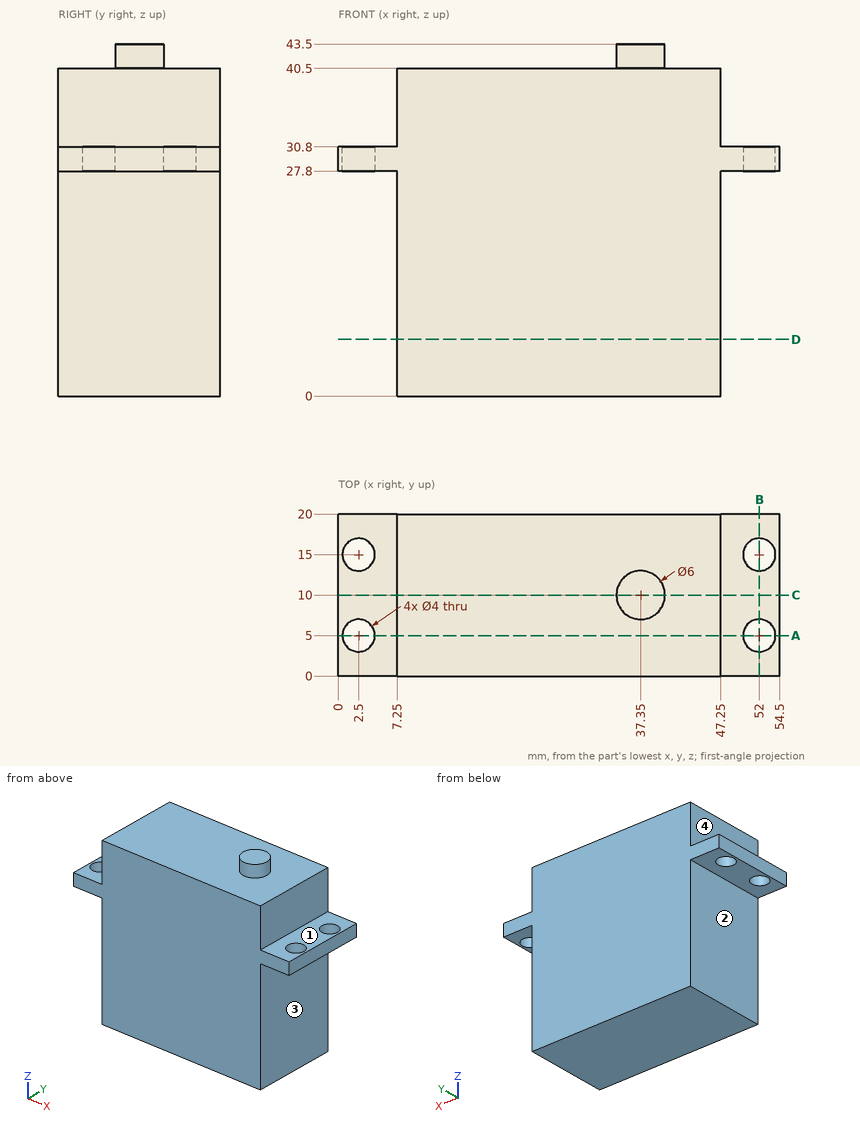
Could you check a few things on this drawing? It's one solid part, dimensions in mm from its lowest x, y, z. A direction names the side the tool comes from. Give positions to 0.01 mm unless a question says otherwise; leave off trailing zeros. Write each loop counter-clockwise with the first axis right and the second up, starting at its lowest first coordinate (ties: lowest second). Pieces come first, ordered by that corner, then holes. Notation, with made-up numbers: (39.5, 88) - (94.5, 88) arc R14 ccw to (94.5, 115) - close; hole circle Ø1 at (44.5, 70.5). An arc over 180 degrees is marked (long way). Use CSV: the item, a comma, the result in double quotes. Start each with the question number.
Item 1: I want a section at D-D, the plane z = 7. Please give me the cut outline in (x, y), then the cut area to 3 significant figures.
Item 2: If I drill on line 1 along Y through (x, z) = (2.5, 28.95); line 2 along Y through (x, z) = (2, 29); line 3 along X through (y, z) = (18, 34.5), over which ranges is the centre line in solid material (lowest first)?
Item 3: I want a section at C-C, the plane y = 10. Please give me the cut outline in (x, z), then the cut area to 3 significant figures.
Item 4: For the marked faces 1, 2, 3 and 4, which set-ups out of +Z, -Z, +X, -X, +Y, -Y let a thin tool reach every point of the face, with its end or its side?
Item 5: I want a section at A-A, the plane y = 5. Please give me the cut outline in (x, z).
Item 6: I'm going to push flat-ended pins straight in: pin 1 (3.5 mm diameter, centred on x = 52, y = 15, fed in from -Z); pin 2 (2 mm diameter, centred on y = 4, z = 17, fed in from -X); pin 3 (5 mm diameter, centred on x = 27, y = 14.5, fed in from +Z); pin 4 (4.5 mm diameter, centred on x = 2.5, y = 15, fed in from -Z). Where does each tip first touch, or does it pass through?
Item 7: I want a section at B-B, the plane x = 52. Please give me the cut outline in (y, z), then the cut area to 3 significant figures.
Findings:
1,outline,"(7.25, 0) - (47.25, 0) - (47.25, 20) - (7.25, 20) - close"
1,area,"800 mm2"
2,line 1,"y = 0 to 3, 7 to 13, 17 to 20"
2,line 2,"y = 0 to 3.06, 6.94 to 13.06, 16.94 to 20"
2,line 3,"x = 7.25 to 47.25"
3,outline,"(0, 27.8) - (7.25, 27.8) - (7.25, 0) - (47.25, 0) - (47.25, 27.8) - (54.5, 27.8) - (54.5, 30.8) - (47.25, 30.8) - (47.25, 40.5) - (40.35, 40.5) - (40.35, 43.5) - (34.35, 43.5) - (34.35, 40.5) - (7.25, 40.5) - (7.25, 30.8) - (0, 30.8) - close"
3,area,"1,680 mm2"
4,face 1,"+Z, +X, +Y, -Y"
4,face 2,"-Z, -X, +Y, -Y"
4,face 3,"-Z, +X, +Y, -Y"
4,face 4,"+Z, -X, +Y, -Y"
5,outline,"(0, 27.8) - (0.5, 27.8) - (0.5, 30.8) - (0, 30.8) - close; (4.5, 27.8) - (7.25, 27.8) - (7.25, 0) - (47.25, 0) - (47.25, 27.8) - (50, 27.8) - (50, 30.8) - (47.25, 30.8) - (47.25, 40.5) - (7.25, 40.5) - (7.25, 30.8) - (4.5, 30.8) - close; (54, 27.8) - (54.5, 27.8) - (54.5, 30.8) - (54, 30.8) - close"
6,pin 1,"passes through"
6,pin 2,"stops at x = 7.25"
6,pin 3,"stops at z = 40.5"
6,pin 4,"stops at z = 27.8"
7,outline,"(0, 27.8) - (3, 27.8) - (3, 30.8) - (0, 30.8) - close; (7, 27.8) - (13, 27.8) - (13, 30.8) - (7, 30.8) - close; (17, 27.8) - (20, 27.8) - (20, 30.8) - (17, 30.8) - close"
7,area,"36.0 mm2"
